```python
from build123d import *

# Parameters (mm, degrees)
ESQUISSE1_R             = 1.65
BOSS_EXTRU_1_DEPTH      = 8
ESQUISSE2_W             = 3.2
ESQUISSE2_H             = 2.278115777
BOSS_EXTRU_2_DEPTH      = 4.2
ESQUISSE3_R             = 0.9
BOSS_EXTRU_3_DEPTH      = 2.3
ESQUISSE4_R             = 1.97
BOSS_EXTRU_4_DEPTH      = 5.32
ENL_V_START             = -5.32
ENL_V_MAT_EXTRU_2_DEPTH = 5.32
BOSS_EXTRU_5_DEPTH      = 0.1
BOSS_EXTRU_6_DEPTH      = 8
BOSS_EXTRU_7_START      = 0.1
BOSS_EXTRU_7_DEPTH      = 0.1


with BuildPart() as part:
    # Esquisse1 → Boss.-Extru.1 (new body)
    with BuildSketch(Plane.XY):
        Circle(ESQUISSE1_R)
    extrude(amount=BOSS_EXTRU_1_DEPTH)

    # Esquisse2 → Boss.-Extru.2 (add)
    with BuildSketch(Plane(origin=(0, 0, 0), x_dir=(-1, 0, 0), z_dir=(0, 0, -1))):
        with Locations((0, -1.011435459)):
            Rectangle(ESQUISSE2_W, ESQUISSE2_H)
    extrude(amount=-BOSS_EXTRU_2_DEPTH)

    # Esquisse3 → Boss.-Extru.3 (add)
    with BuildSketch(Plane.XY.offset(8)):
        Circle(ESQUISSE3_R)
    extrude(amount=BOSS_EXTRU_3_DEPTH)

    # Esquisse4 → Boss.-Extru.4 (add)
    with BuildSketch(Plane.XY.offset(10.3)):
        Circle(ESQUISSE4_R)
    extrude(amount=BOSS_EXTRU_4_DEPTH)

    # Esquisse6 → Enlèv. mat.-Extru.2 (cut)
    with BuildSketch(Plane.XY.offset(15.62).offset(ENL_V_START)):
        with BuildLine():
            Line((-1.97, 0), (-1.25, 0))
            ThreePointArc((-1.25, 0), (0, 1.25), (1.25, 0))
            Line((1.25, 0), (1.97, 0))
            ThreePointArc((1.97, 0), (0, 1.97), (-1.97, 0))
        make_face()
    extrude(amount=ENL_V_MAT_EXTRU_2_DEPTH, mode=Mode.SUBTRACT)

    # Esquisse7 → Boss.-Extru.5 (add)
    with BuildSketch(Plane.XZ.offset(2.150493347)):
        with BuildLine():
            Line((1.6, 0), (0.3, 0))
            Line((0.3, 0), (0.3, 4.2))
            ThreePointArc((0.3, 4.2), (0.446446609, 4.553553391), (0.8, 4.7))
            Line((0.8, 4.7), (1.1, 4.7))
            ThreePointArc((1.1, 4.7), (1.453553391, 4.553553391), (1.6, 4.2))
            Line((1.6, 4.2), (1.6, 0))
        make_face()
        with BuildLine():
            Line((-1.6, 0), (-0.3, 0))
            Line((-0.3, 0), (-0.3, 4.2))
            ThreePointArc((-0.3, 4.2), (-0.446446609, 4.553553391), (-0.8, 4.7))
            Line((-0.8, 4.7), (-1.1, 4.7))
            ThreePointArc((-1.1, 4.7), (-1.453553391, 4.553553391), (-1.6, 4.2))
            Line((-1.6, 4.2), (-1.6, 0))
        make_face()
    extrude(amount=BOSS_EXTRU_5_DEPTH)

    # Esquisse8 → Boss.-Extru.6 (add)
    with BuildSketch(Plane(origin=(0, 0, 0), x_dir=(-1, 0, 0), z_dir=(0, 0, -1))):
        with BuildLine():
            Line((-1.65, 0), (-1.65, -2.150493347))
            Line((-1.65, -2.150493347), (1.6, -2.150493347))
            Line((1.6, -2.150493347), (1.61, -2.150493347))
            Line((1.61, -2.150493347), (1.65, 0))
            ThreePointArc((1.65, 0), (0, 1.686495035), (-1.65, 0))
        make_face()
    extrude(amount=-BOSS_EXTRU_6_DEPTH)

    # Esquisse9 → Boss.-Extru.7 (add)
    with BuildSketch(Plane(origin=(0, 0, 0), x_dir=(-1, 0, 0), z_dir=(0, 0, -1)).offset(BOSS_EXTRU_7_START)):
        with BuildLine():
            Line((-1.25, 0), (-1.25, -2.150493347))
            Line((-1.25, -2.150493347), (-1.65, -2.150493347))
            Line((-1.65, -2.150493347), (-1.650394869, 0.036100167))
            ThreePointArc((-1.650394869, 0.036100167), (0.018054459, 1.686697641), (1.65, 0))
            Line((1.65, 0), (1.6, -2.150493347))
            Line((1.6, -2.150493347), (1.25, -2.150493347))
            Line((1.25, -2.150493347), (1.25, 0))
            ThreePointArc((1.25, 0), (0, 1.25), (-1.25, 0))
        make_face()
    extrude(amount=-BOSS_EXTRU_7_DEPTH)


solid = part.part
```
Check sheet for the modelled part. Datum: model origin and axes. Units: mm. A direction names the side the tool comes from. Coordinates: 2 decimals unless noted, no trailing zeros. Order: outer loops, then holes, each group sorted by start corner. A loop starts at its lowest first (then second) coordinate and runs counter-clockwise, first axis right, second up. Notation, with made-up numbers: (39.25, -27.5) -> (81.25, -27.5) arc R7 ccw to (81.25, -15.5) -> close; hole circle Ø5 at (9, 66.25). An arc over 180 degrees is marked (long way). Write each question's results on one line, items separated by ' | '. Start each with the question number.
1) Material ranges on line 1 along Z through (x, y) = (-1, -0.9); line 2 along Z through (x, y) = (-1.55, -1); line 3 along Z through (x, y) = (0.25, -0.4), recorded low to high.
2) Section check D-D (z = 6.5). Enter the section's corners in (x, y).
3) Set-up check for faces 1 (the face through (0, 0, 15.62)), 2 (the face through (1.65, -1, 4)), 3 (the face through (-0.03, 1.25, 12.92)), 4 (the face through (-0.04, -1.97, 12.92)), 5 (the face through (0, -1.1, 10.3)): record each of +Z, -Z, +X, -X, +Y, -Y from which the full face is reachable in a straight line by a thin tool's end or side.
4) Draft check along Z on faces 6 (the face through (-1, 1, -0.1)), 7 (the face through (0.86, 0.27, 9.13)), 8 (the face through (-1, -2.25, 2)). Enter one of: pulls with the +Z half, pulls with the -Z half, needs draft (parallel to the pull), parting line crosses it, or undercut.
5) Depth check by flat-ended pin: pin 1 (1.5 mm diameter, centred on x = -0.5, z = 10, fed in from -Y); pin 2 (1.7 mm diameter, centred on y = -1, z = 4, fed in from +X); pin 3 (1.5 mm diameter, centred on y = 0.5, z = 2.5, fed in from +X). Enter the tip coordinate at first touch or a pass-through.
Checked values:
1) line 1: 0 to 8, 10.3 to 15.62 | line 2: -0.1 to 8, 10.3 to 15.62 | line 3: 0 to 15.62
2) outline: (-1.65, -0.06) -> (-1.61, -2.15) -> (1.65, -2.15) -> (1.65, 0) arc R1.65 ccw (long way) to (-1.65, 0) arc R1.65 ccw to start
3) face 1: +Z, +X, -X, +Y, -Y | face 2: -Z, +X, +Y, -Y | face 3: +Z, +Y | face 4: +Z, -Y | face 5: none
4) face 6: pulls with the -Z half | face 7: undercut | face 8: needs draft
5) pin 1: y = -1.97 | pin 2: x = 1.65 | pin 3: x = 1.65
